```python
from build123d import *

# Parameters (mm, degrees)
BOSS_EXTRUDE1_DEPTH = 16
SKETCH4_R           = 4.5
BOSS_EXTRUDE2_DEPTH = 4
SKETCH2_R           = 1.65
CUT_EXTRUDE1_DEPTH  = 10
CUT_EXTRUDE2_START  = -4
CUT_EXTRUDE2_DEPTH  = 3.2
CHAMFER1_SIZE       = 0.3
CUT_EXTRUDE3_DEPTH  = 10


with BuildPart() as part:
    # Sketch1 → Boss-Extrude1 (new body)
    with BuildSketch(Plane.XY):
        with BuildLine():
            Line((8, -6.800735254), (8, -10.5))
            Line((8, -10.5), (15, -10.5))
            Line((15, -10.5), (15, 0))
            ThreePointArc((15, 0), (0, 15), (-15, 0))
            Line((-15, 0), (-15, -10.5))
            Line((-15, -10.5), (-8, -10.5))
            Line((-8, -10.5), (-8, -6.800735254))
            ThreePointArc((-8, -6.800735254), (0, 10.5), (8, -6.800735254))
        make_face()
    extrude(amount=BOSS_EXTRUDE1_DEPTH)

    # Sketch4 → Boss-Extrude2 (add)
    with BuildSketch(Plane.XZ.offset(10.5)):
        with Locations((14, 8)):
            Circle(SKETCH4_R)
    boss_extrude2 = extrude(amount=-BOSS_EXTRUDE2_DEPTH)

    # Sketch2 → Cut-Extrude1 (cut)
    with BuildSketch(Plane.XZ.offset(10.5)):
        with Locations((13, 8)):
            Circle(SKETCH2_R)
    cut_extrude1 = extrude(amount=-CUT_EXTRUDE1_DEPTH, mode=Mode.SUBTRACT)

    # Sketch3 → Cut-Extrude2 (cut)
    with BuildSketch(Plane.XZ.offset(10.5).offset(CUT_EXTRUDE2_START)):
        Polygon((10.2, 9.616580754), (10.2, 9.916580754), (13, 11.533161507), (17.758039714, 11.533161507), (17.758039714, 11.233161507), (17.758039714, 4.766838493), (13, 4.766838493), (10.2, 6.383419246), align=None)
    cut_extrude2 = extrude(amount=-CUT_EXTRUDE2_DEPTH, mode=Mode.SUBTRACT)

    # Mirror1: Boss-Extrude2, Cut-Extrude1, Cut-Extrude2 across plane
    add(boss_extrude2.mirror(Plane(origin=(0, 0, 0), x_dir=(0, 0, 1), z_dir=(1, 0, 0))))
    add(cut_extrude1.mirror(Plane(origin=(0, 0, 0), x_dir=(0, 0, 1), z_dir=(1, 0, 0))), mode=Mode.SUBTRACT)
    add(cut_extrude2.mirror(Plane(origin=(0, 0, 0), x_dir=(0, 0, 1), z_dir=(1, 0, 0))), mode=Mode.SUBTRACT)

    # Chamfer1
    chamfer1_edges = [part.edges().sort_by_distance(p)[0] for p in [
        (-15, -5.25, 0),
        (0, 15, 0),
        (15, -5.25, 0),
        (11.5, -10.5, 0),
        (8, -8.650367627, 0),
        (0, 10.5, 0),
        (-8, -8.650367627, 0),
        (-11.5, -10.5, 0),
    ]]
    chamfer(chamfer1_edges, length=CHAMFER1_SIZE)

    # Sketch5 → Cut-Extrude3 (cut)
    with BuildSketch(Plane.XZ.offset(10.5)):
        Polygon((-13, 8), (-11.833273811, 9.166726189), (-12.636547622, 9.97), (-13.363452378, 9.97), (-14.166726189, 9.166726189), align=None)
        Polygon((13, 8), (14.166726189, 9.166726189), (13.363452378, 9.97), (12.636547622, 9.97), (11.833273811, 9.166726189), align=None)
    extrude(amount=-CUT_EXTRUDE3_DEPTH, mode=Mode.SUBTRACT)


solid = part.part
```
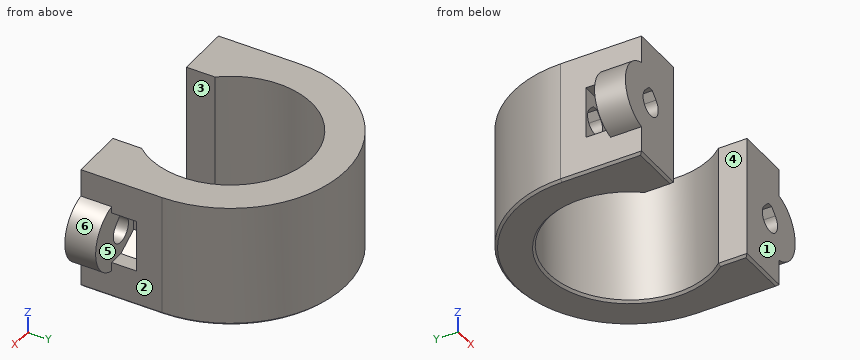
CAD build for the part. Positions are in the model's coordinates, mm. Face numbers are marked on the shaded views. A direction names the side the tool comes from. Give positions to 0.01 mm unless a question says otherwise; leave off trailing zeros. Write each loop counter-clockwise with the first axis right and the second up, starting at its lowest first coordinate (ties: lowest second). Pieces come first, ordered by that corner, then holes. Notation, with made-up numbers: (4, -16.5) -> (23, -16.5) arc R9 cw to (23, -7.5) -> close; hole circle Ø1 at (-17.75, 14). An arc over 180 degrees is marked (long way). Write each question's results on one line, items separated by ' | '.
1. Cut at B-B, the plane y = -8.5. Write the cut outline in (x, z).
Geometry check:
outline: (-15, 0.3) -> (-14.7, 0) -> (-8.3, 0) -> (-8, 0.3) -> (-8, 16) -> (-15, 16) -> (-15, 12.39) arc R4.5 ccw to (-15, 3.61) -> close; (8, 0.3) -> (8.3, 0) -> (14.7, 0) -> (15, 0.3) -> (15, 3.61) arc R4.5 ccw to (15, 12.39) -> (15, 16) -> (8, 16) -> close; hole (-14.17, 9.17) arc R1.65 ccw (long way) to (-11.83, 9.17) -> (-12.64, 9.97) -> (-13.36, 9.97) -> close; hole (11.83, 9.17) arc R1.65 ccw (long way) to (14.17, 9.17) -> (13.36, 9.97) -> (12.64, 9.97) -> close
2. Two-plate mould, pull along X, no slides. Class the marked faces 1, 2, 3 and 4: pulls with the +X half, pulls with the -X half, needs draft (parallel to the pull), parting line crosses it, or undercut.
Geometry check:
face 1: needs draft | face 2: pulls with the +X half | face 3: undercut | face 4: undercut
3. Cut at C-C, the plane z = 13.25. Write the cut outline in (x, y).
Geometry check:
outline: (-15, -10.5) -> (-8, -10.5) -> (-8, -6.8) arc R10.5 cw (long way) to (8, -6.8) -> (8, -10.5) -> (15, -10.5) -> (15, 0) arc R15 ccw to (-15, 0) -> close
4. Cut at A-A, the plane z = 8. Give the number of separate pieces and of enclosed holes in the cut face, then the cut area to 3 significant figures.
Geometry check:
separate pieces: 3 | enclosed holes: 0 | area: 256 mm²
5. Wall check: probe 1 along X at (y, z) = (-9.45, 8); probe 2 along Z at (x, y) = (13, -2.25); probe 3 along X at (y, z) = (-1.8, 8). Give the ranges that are in metal, low to high. Write a range as [from, to].
Geometry check:
probe 1: [-18.5, -14.65], [-11.35, -8], [8, 11.35], [14.65, 18.5] | probe 2: [0, 6.35], [9.97, 16] | probe 3: [-15, -14.65], [-11.35, -10.34], [10.34, 11.35], [14.65, 15]
6. Which spindle directions (+Z, -Z, +X, -X, +Y, -Y) get a long thin tool onto all of the face, cutting with end or side? Do the marked faces 5 and 6. Say none if no direction does.
Geometry check:
face 5: +X | face 6: +X, +Y, -Y
7. Cut at D-D, the plane x = 0. Write the cut outline in (y, z).
Geometry check:
outline: (10.5, 0.3) -> (10.8, 0) -> (14.7, 0) -> (15, 0.3) -> (15, 16) -> (10.5, 16) -> close
8. Drop flat-ended pins along their axis: P1, Ø2.5, axis at y = -4.5, z = 8, coming from the -X side; P2, Ø1.8, axis at y = -9, z = 5, coming from the -X side; P3, Ø6.5, axis at x = -13.5, z = 7.5, coming from the +Y side. Give the stop position or say it passes through.
Geometry check:
P1: x = -15 | P2: x = -17.98 | P3: y = 10.95
